Check sheet for the drawn part. Datum: minimum x, y, z corner. Units: mm. A direction names the side the tool comes from. Round coordinates to 2 decimals unless told otherwise and drop trailing zeros. Order: outer loops, then holes, each group sorted by start corner. A loop starts at its lowest first (then second) coordinate and runs counter-clockwise, first axis right, second up. Notation, with made-up numbers: M 59,6 L 81,6 A23 ccw 81,43 Z; hole C 58,45.5 d8. An arc over 180 degrees is marked long. Use one line per item in the form item = value. Start each with the question number.
Item 1: Cross-section at A-A on z = 2. Enter the section's corners in (x, y), then the cut area to 3 significant figures.
Item 2: Cross-section at B-B on x = 6.5. Enter the section's corners in (y, z).
Item 3: Thickness scan on probe 1 along Z at (x, y) = (4.75, 2); probe 2 along X at (y, z) = (1.8, 2.55). Record the ranges inside material, lowest first. Write a range as [from, to].
Item 4: Tool access check on the marked faces 1 and 2. Record the directions out of +Z, -Z, +X, -X, +Y, -Y that give a thin tool (end or side, any length) a straight path to the whole face; none if there is none.
Item 5: Go/stop test with a flat-tipped pin: pin 1 Ø1 at (y, z) = (2.5, 2) entering from -X. Record where the tip stops, or that it passes through.
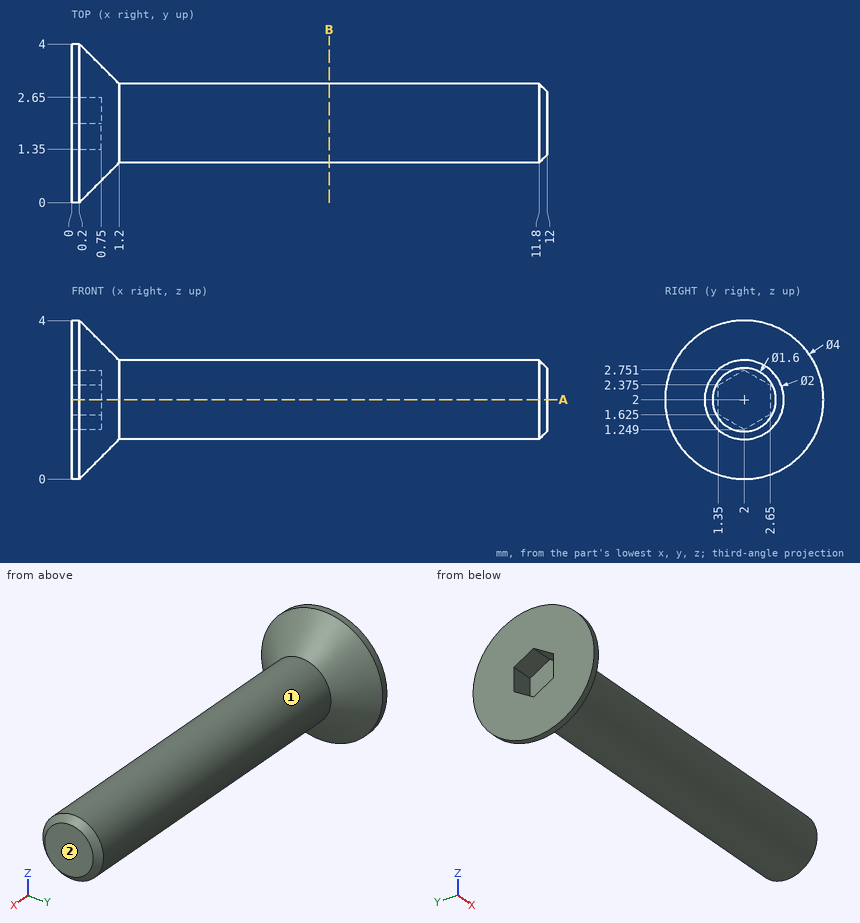
Output values:
q1.outline = M 0,0 L 0.2,0 L 1.2,1 L 11.8,1 L 12,1.2 L 12,2.8 L 11.8,3 L 1.2,3 L 0.2,4 L 0,4 L 0,2.65 L 0.75,2.65 L 0.75,1.35 L 0,1.35 Z
q1.area = 24.4 mm2
q2.outline = C 2,2 d2
q3.probe_1 = [1, 3]
q3.probe_2 = [0.75, 12]
q4.face_1 = +X
q4.face_2 = +Z, -Z, +X, +Y, -Y
q5.pin_1 = 0
